Autodesk Inventor part; units mm, degrees
ref_plane "YZ Plane" through (0, 0, 0) normal (1, 0, 0) x (0, 1, 0)
ref_plane "XZ Plane" through (0, 0, 0) normal (0, 1, 0) x (-1, 0, 0)
ref_plane "XY Plane" through (0, 0, 0) normal (0, 0, 1) x (1, 0, 0)
sketch "Эскиз1" plane through (0, 0, 0) normal (0, 1, 0) x (-1, 0, 0)
  line L0 (4.5, 0) -> (45.5, 0)
  line L1 (50, 4.5) -> (50, 45.5)
  line L2 (45.5, 50) -> (4.5, 50)
  line L3 (0, 45.5) -> (0, 4.5)
  arc A0 (50, 45.5) -> (45.5, 50) centre (45.5, 45.5) ccw
  arc A1 (45.5, 0) -> (50, 4.5) centre (45.5, 4.5) ccw
  arc A2 (4.5, 50) -> (0, 45.5) centre (4.5, 45.5) ccw
  arc A3 (0, 4.5) -> (4.5, 0) centre (4.5, 4.5) ccw
  point P0 (0, 0)
  point P1 (50, 50)
  point P2 (50, 0)
  point P3 (0, 50)
  dimension "d0" = 50
  dimension "d1" = 50
  dimension "d2" = 4.5
  dimension "d3" = 4.5
  dimension "d4" = 4.5
  dimension "d5" = 4.5
extrude "Выдавливание1" add sketch "Эскиз1" along normal blind 2
sketch "Эскиз2" plane through (0, 2, 0) normal (0, 1, 0) x (1, 0, 0)
  line L0 (-50, -4.5) -> (-50, -45.5)
  line L1 (-50, -25) -> (0, -25)
  line L2 (0, -45.5) -> (0, -4.5)
  circle A0 centre (-25, -25) radius 3
  arc A1 (-45.5, 0) -> (-50, -4.5) centre (-45.5, -4.5) ccw
  line L3 (-50, -4.5) -> (-50, -45.5)
  arc A2 (-50, -45.5) -> (-45.5, -50) centre (-45.5, -45.5) ccw
  line L4 (-45.5, -50) -> (-4.5, -50)
  arc A3 (-4.5, -50) -> (0, -45.5) centre (-4.5, -45.5) ccw
  line L5 (0, -45.5) -> (0, -4.5)
  arc A4 (0, -4.5) -> (-4.5, 0) centre (-4.5, -4.5) ccw
  line L6 (-4.5, 0) -> (-45.5, 0)
  line L7 (-30, -32) -> (-20, -32)
  line L8 (-18, -30) -> (-18, -20)
  line L9 (-20, -18) -> (-30, -18)
  line L10 (-32, -20) -> (-32, -30)
  line L11 (-32, -32) -> (-18, -18) construction
  line L12 (-18, -32) -> (-32, -18) construction
  arc A5 (-30, -18) -> (-32, -20) centre (-30, -20) ccw
  arc A6 (-32, -30) -> (-30, -32) centre (-30, -30) ccw
  arc A7 (-20, -32) -> (-18, -30) centre (-20, -30) ccw
  arc A8 (-18, -20) -> (-20, -18) centre (-20, -20) ccw
  point P0 (0, 0)
  dimension "d8" = 6
  dimension "d9" = 14
  dimension "d10" = 14
  dimension "d11" = 2
  dimension "d12" = 2
extrude "Выдавливание2" add sketch "Эскиз2" along normal blind 5 contours L10 A5 L9 A8 L8 L1 A0 | L1 A0 L8 A7 L7 A6 L10
chamfer "Фаска1" distance 2 angle 45 8 edges at (-25, 2, 32) (-31.4142, 2, 31.4142) (-32, 2, 25) (-31.4142, 2, 18.5858) (-25, 2, 18) (-18.5858, 2, 18.5858) (-18, 2, 25) (-18.5858, 2, 31.4142)
extrude "Выдавливание3" cut sketch "Эскиз2" against normal blind 5 contours A0 L1 | L1 A0
thread "Резьба1"
sketch "Эскиз3" plane through (0, 2, 0) normal (0, 1, 0) x (1, 0, 0)
  arc A0 (-45.5, 0) -> (-50, -4.5) centre (-45.5, -4.5) ccw
  line L0 (-50, -4.5) -> (-50, -45.5)
  arc A1 (-50, -45.5) -> (-45.5, -50) centre (-45.5, -45.5) ccw
  line L1 (-45.5, -50) -> (-4.5, -50)
  arc A2 (-4.5, -50) -> (0, -45.5) centre (-4.5, -45.5) ccw
  line L2 (0, -45.5) -> (0, -4.5)
  arc A3 (0, -4.5) -> (-4.5, 0) centre (-4.5, -4.5) ccw
  line L3 (-4.5, 0) -> (-45.5, 0)
  line L4 (-30, -34) -> (-20, -34)
  arc A4 (-34, -30) -> (-30, -34) centre (-30, -30) ccw
  line L5 (-34, -20) -> (-34, -30)
  arc A5 (-30, -16) -> (-34, -20) centre (-30, -20) ccw
  line L6 (-20, -16) -> (-30, -16)
  arc A6 (-16, -20) -> (-20, -16) centre (-20, -20) ccw
  line L7 (-16, -30) -> (-16, -20)
  arc A7 (-20, -34) -> (-16, -30) centre (-20, -30) ccw
  line L8 (-1, -4.5) -> (-1, -45.5)
  arc A8 (-4.5, -49) -> (-1, -45.5) centre (-4.5, -45.5) ccw
  line L9 (-4.5, -49) -> (-45.5, -49)
  arc A9 (-49, -45.5) -> (-45.5, -49) centre (-45.5, -45.5) ccw
  line L10 (-49, -45.5) -> (-49, -4.5)
  arc A10 (-45.5, -1) -> (-49, -4.5) centre (-45.5, -4.5) ccw
  line L11 (-45.5, -1) -> (-4.5, -1)
  arc A11 (-1, -4.5) -> (-4.5, -1) centre (-4.5, -4.5) ccw
  point P0 (0, 0)
  dimension "d22" = 1
extrude "Выдавливание4" cut sketch "Эскиз3" against normal blind 10 contours L3 A3 L2 A2 L1 A1 L0 A0
properties part number "Bottom_contact" material "Сталь нержавеющая AISI 202"
Part model, mm, in its own coordinate system. A direction names the side the tool comes from. Coordinates: 2 decimals unless noted, no trailing zeros. Order: outer loops, then holes, each group sorted by start corner. A loop starts at its lowest first (then second) coordinate and runs counter-clockwise, first axis right, second up. Notation, with made-up numbers: (15, -3.75) -> (20, -3.75) arc R28 cw to (20, 24.25) -> close; hole circle Ø6 at (41, 2.5). An arc over 180 degrees is marked (long way). Put each result on its own line as item: value. Start each with the question number.
(1) Band-saw the part on D-D (y = 5). Give the cut face in (x, z), then the cut area to 3 significant figures.
(2) Band-saw the part on A-A (z = 25). Give the cut face in (x, y), then the cut area to 3 significant figures.
(3) Mould opens along X. For faces 1 (the face through (-33, 3, 25)), 2 (the face through (-25, 1, 1)), 3 (the face through (-28, 4, 25)) say: pulls with the +X half, pulls with the -X half, needs draft (parallel to the pull), parting line crosses it, or undercut.
(4) Probe line 1 along X through (y, z) = (5.75, 25); line 2 along Z through (x, y) = (-25, 1.75); line 3 along Z through (x, y) = (-25, 4.25). List the from-to ranges inside material, lowest first. Write a range as [from, to].
(5) Which spindle directions (+Z, -Z, +X, -X, +Y, -Y) get a long thin tool onto all of the face, cutting with end or side? Do faces 4 (the face through (-25, 5, 18)), 5 (the face through (-31.4, 5.48, 31.43)), 6 (the face through (-18.57, 5.48, 31.4)). Say none if no direction does.
(6) Pin check, flat tips, straight feed: pin 1 Ø2.5 at (y, z) = (5, 24.5) entering from +X; pin 2 Ø1 at (x, y) = (-21, 3) entering from -Z; pin 3 Ø2.5 at (x, y) = (-23.5, 6) entering from -Z; pin 4 Ø2 at (x, z) = (-32, 12) entering from -Y. Stop position of each tip, or through.
(7) Band-saw the part on B-B (y = 1.25). Give the cut face in (x, z).
(8) Band-saw the part on C-C (x = -25). Give the cut face in (y, z).
Determined:
1. outline: (-32, 20) arc R2 ccw to (-30, 18) -> (-20, 18) arc R2 ccw to (-18, 20) -> (-18, 30) arc R2 ccw to (-20, 32) -> (-30, 32) arc R2 ccw to (-32, 30) -> close; hole circle Ø6 at (-25, 25)
1. area: 164 mm²
2. outline: (-49, 0) -> (-28, 0) -> (-28, 7) -> (-32, 7) -> (-32, 4) -> (-34, 2) -> (-49, 2) -> close; (-22, 0) -> (-1, 0) -> (-1, 2) -> (-16, 2) -> (-18, 4) -> (-18, 7) -> (-22, 7) -> close
2. area: 128 mm²
3. face 1: pulls with the -X half
3. face 2: needs draft
3. face 3: undercut
4. line 1: x = [-32, -28], [-22, -18]
4. line 2: z = [1, 22], [28, 49]
4. line 3: z = [18, 22], [28, 32]
5. face 4: -Z, +X, -X, +Y
5. face 5: +Z, -X, +Y
5. face 6: +Z, +X, +Y
6. pin 1: stops at x = -17.75
6. pin 2: stops at z = 16.5
6. pin 3: stops at z = 18
6. pin 4: stops at y = 0
7. outline: (-49, 4.5) arc R3.5 ccw to (-45.5, 1) -> (-4.5, 1) arc R3.5 ccw to (-1, 4.5) -> (-1, 45.5) arc R3.5 ccw to (-4.5, 49) -> (-45.5, 49) arc R3.5 ccw to (-49, 45.5) -> close; hole circle Ø6 at (-25, 25)
8. outline: (0, 1) -> (2, 1) -> (2, 16) -> (4, 18) -> (7, 18) -> (7, 22) -> (0, 22) -> close; (0, 28) -> (7, 28) -> (7, 32) -> (4, 32) -> (2, 34) -> (2, 49) -> (0, 49) -> close
